Geometry: final body of the model. Coordinates: model frame, mm. A direction names the side the tool comes from. Give positions to 0.01 mm unless a question says otherwise; leave off trailing zeros. Write each loop counter-clockwise with the first axis right and the second up, starting at its lowest first coordinate (ties: lowest second). Pieces come first, ordered by that corner, then holes. Notation, with made-up numbers: M -3.75,29 L 24.25,29 A14 ccw 24.25,34 Z; hole C 3.25,-1.5 d3. An arc over 180 degrees is marked long. Answer as a JSON object with one key per item and string values.
Autodesk Inventor part; units mm, degrees
ref_plane "YZ Plane" through (0, 0, 0) normal (1, 0, 0) x (0, 1, 0)
ref_plane "XZ Plane" through (0, 0, 0) normal (0, 1, 0) x (-1, 0, 0)
ref_plane "XY Plane" through (0, 0, 0) normal (0, 0, 1) x (1, 0, 0)
sketch "Sketch1" plane through (0, 0, 0) normal (0, 1, 0) x (-1, 0, 0)
  circle A0 centre (0, 0) radius 2.85
  dimension "d0" = 5.7
extrude "Extrusion1" add sketch "Sketch1" along normal blind 2.2
sketch "Sketch2" plane through (0, 0, 0) normal (0, -1, 0) x (1, 0, 0)
  circle A0 centre (0, 0) radius 1.5
  dimension "d3" = 3
extrude "Extrusion2" add sketch "Sketch2" along normal blind 5.8
fillet "Fillet1" radius 0.8 1 edges at (2.85, 2.2, 0)
sketch "Sketch3" plane through (0, 2.2, 0) normal (0, 1, 0) x (1, 0, 0)
  line L0 (0.4, -1.6) -> (-0.4, -1.6)
  line L1 (-0.4, -1.6) -> (-0.4, 1.6)
  line L2 (-0.4, 1.6) -> (0.4, 1.6)
  line L3 (0.4, 1.6) -> (0.4, -1.6)
  line L4 (0.4, -1.6) -> (-0.4, 1.6) construction
  line L5 (-0.4, -1.6) -> (0.4, 1.6) construction
  line L6 (1.6, 0.4) -> (-1.6, 0.4)
  line L7 (-1.6, 0.4) -> (-1.6, -0.4)
  line L8 (-1.6, -0.4) -> (1.6, -0.4)
  line L9 (1.6, -0.4) -> (1.6, 0.4)
  circle A0 centre (0, 0) radius 1.5
  line L10 (1.6, 0.4) -> (-1.6, -0.4) construction
  line L11 (-1.6, 0.4) -> (1.6, -0.4) construction
  point P0 (0.4, 0.4)
  point P1 (-0.4, 0.4)
  point P2 (-0.4, -0.4)
  point P3 (0.4, -0.4)
  dimension "d7" = 0.8
  dimension "d8" = 0.8
  dimension "d9" = 3.2
  dimension "d10" = 3.2
extrude "Extrusion3" cut sketch "Sketch3" against normal blind 1 contours L0 L1 A0 L3 | A0 L1 L8 L3 | L8 L1 L6 L3 | L3 L6 A0 L8 | A0 L6 L9 L8 | L8 A0 L6 L1 | L8 L7 L6 A0 | L6 L1 A0 L3 | A0 L1 L2 L3
chamfer "Chamfer1" distance 0.5 angle 45 1 edges at (-1.5, -5.8, 0)
thread "Thread1"
properties part number "support_screw"
1) Pull-direction query (Z, two-part tool) for faces 4 (the flat face through (0.4, 2, 1)), 5 (the flat face through (-1.2, 0, -1.2)), 6 (the cylindrical face through (2.262, 0.69, 1.734)); classes: pulls with the +Z half, pulls with the -Z half, needs draft (parallel to the pull), parting line crosses it, or undercut.
Geometry check:
{"face 4": "undercut", "face 5": "needs draft", "face 6": "parting line crosses it"}
2) Cut plane C-C on y = -4.25. Return loops of the section in (x, z), and give its area (3 significant figures).
Geometry check:
{"outline": "C 0,0 d3", "area": "7.07 mm2"}
3) Cut plane A-A on x = 0. Return loops of the section in (y, z), and give its area (3 significant figures).
Geometry check:
{"outline": "M -5.8,-1 L -5.3,-1.5 L 0,-1.5 L 0,-2.85 L 1.4,-2.85 A0.8 ccw 2.2,-2.05 L 2.2,-1.6 L 1.2,-1.6 L 1.2,1.6 L 2.2,1.6 L 2.2,2.05 A0.8 ccw 1.4,2.85 L 0,2.85 L 0,1.5 L -5.3,1.5 L -5.8,1 Z", "area": "26.2 mm2"}
4) Contact query for flat-ended pins moving along their axis: P1, Ø0.5, axis at y = 1.5, z = -1, coming from the +X side; P2, Ø1.1, axis at x = -1, y = 2, coming from the -Z side; P3, Ø1.5, axis at x = -0.5, y = -5, coming from the +Z side. Output: stop coordinate, or through.
Geometry check:
{"P1": "stops at x = 2.75", "P2": "stops at z = -2.76", "P3": "stops at z = 1.5"}
5) Cut plane B-B on z = 0. Return loops of the section in (x, y), and give its area (3 significant figures).
Geometry check:
{"outline": "M -2.85,0 L -1.5,0 L -1.5,-5.3 L -1,-5.8 L 1,-5.8 L 1.5,-5.3 L 1.5,0 L 2.85,0 L 2.85,1.4 A0.8 ccw 2.05,2.2 L 1.6,2.2 L 1.6,1.2 L -1.6,1.2 L -1.6,2.2 L -2.05,2.2 A0.8 ccw -2.85,1.4 Z", "area": "26.2 mm2"}
6) Line query: line 1 (Z direction, x = -0.5, y = 1.75); line 2 (X direction, y = 2, z = 0.05); line 3 (Y direction, x = 1.4, z = 1.1). Output: solid intervals per line, ascending. Write a range as from..to.
Geometry check:
{"line 1": "z = -2.72..-0.4, 0.4..2.72", "line 2": "x = -2.58..-1.6, 1.6..2.58", "line 3": "y = 0..2.2"}
7) Set-up query: faces 1 (the flat face through (0, -5.8, 0)), 2 (the cylindrical face through (-1.5, -2.61, -0.07)), 3 (the flat face through (-1, 2, 0.4)). Return all of +Z, -Z, +X, -X, +Y, -Y with unobstructed straight access to the full face (end or side cutting, diameter ignored); none if empty.
Geometry check:
{"face 1": "+Z, -Z, +X, -X, -Y", "face 2": "-Y", "face 3": "+Y"}
